```python
from build123d import *

# Parameters (mm, degrees)
SKETCH13_R          = 2.5
SKETCH13_R_2        = 1.5
SKETCH13_W          = 0.45
SKETCH13_H          = 1.7
BOSS_EXTRUDE1_DEPTH = 1.6


with BuildPart() as part:
    # Sketch13 → Boss-Extrude1 (new body)
    # profile 1 of 5: a face of its own
    with BuildSketch(Plane.XY):
        with BuildLine():
            Line((115.98540719, 133.738694526), (115.45540719, 133.738694526))
            ThreePointArc((115.45540719, 133.738694526), (111.919873284, 132.274228432), (110.45540719, 128.738694526))
            Line((110.45540719, 128.738694526), (110.45540719, 123.738694526))
            Line((110.45540719, 123.738694526), (110.45540719, 118.738694526))
            ThreePointArc((110.45540719, 118.738694526), (111.582423844, 115.576416866), (114.45540719, 113.83971504))
            Line((114.45540719, 113.83971504), (114.45540719, 120.238694526))
            Line((114.45540719, 120.238694526), (126.45540719, 120.238694526))
            Line((126.45540719, 120.238694526), (126.45540719, 113.83971504))
            ThreePointArc((126.45540719, 113.83971504), (129.328390536, 115.576416866), (130.45540719, 118.738694526))
            Line((130.45540719, 118.738694526), (130.45540719, 123.738694526))
            Line((130.45540719, 123.738694526), (130.45540719, 128.738694526))
            ThreePointArc((130.45540719, 128.738694526), (128.990941096, 132.274228432), (125.45540719, 133.738694526))
            Line((125.45540719, 133.738694526), (124.92540719, 133.738694526))
            Line((124.92540719, 133.738694526), (124.92540719, 127.388694526))
            Line((124.92540719, 127.388694526), (115.98540719, 127.388694526))
            Line((115.98540719, 127.388694526), (115.98540719, 131.288694526))
            Line((115.98540719, 131.288694526), (115.53540719, 131.288694526))
            Line((115.53540719, 131.288694526), (115.53540719, 132.988694526))
            Line((115.53540719, 132.988694526), (115.98540719, 132.988694526))
            Line((115.98540719, 132.988694526), (115.98540719, 133.738694526))
        make_face()
        with BuildLine():
            ThreePointArc((115.45540719, 123.738694526), (112.95540719, 121.238694526), (110.45540719, 123.738694526))
            ThreePointArc((110.45540719, 123.738694526), (112.95540719, 126.238694526), (115.45540719, 123.738694526))
        make_face(mode=Mode.SUBTRACT)
        with Locations((127.95540719, 123.738694526)):
            Circle(SKETCH13_R, mode=Mode.SUBTRACT)
    # profile 2 of 5: a face of its own
    with BuildSketch(Plane.XY):
        with Locations((112.95540719, 123.738694526)):
            Circle(SKETCH13_R)
        with Locations((112.95540719, 123.738694526)):
            Circle(SKETCH13_R_2, mode=Mode.SUBTRACT)
    # profile 3 of 5: a face of its own
    with BuildSketch(Plane.XY):
        with Locations((127.95540719, 123.738694526)):
            Circle(SKETCH13_R)
        with Locations((127.95540719, 123.738694526)):
            Circle(SKETCH13_R_2, mode=Mode.SUBTRACT)
    # profile 4 of 5: a face of its own
    with BuildSketch(Plane.XY):
        with BuildLine():
            Line((114.45540719, 120.238694526), (114.45540719, 113.83971504))
            ThreePointArc((114.45540719, 113.83971504), (114.95286238, 113.764013761), (115.45540719, 113.738694526))
            Line((115.45540719, 113.738694526), (125.45540719, 113.738694526))
            ThreePointArc((125.45540719, 113.738694526), (125.957952, 113.764013761), (126.45540719, 113.83971504))
            Line((126.45540719, 113.83971504), (126.45540719, 120.238694526))
            Line((126.45540719, 120.238694526), (114.45540719, 120.238694526))
        make_face()
    # profile 5 of 5: a face of its own
    with BuildSketch(Plane.XY):
        with Locations((115.76040719, 132.138694526)):
            Rectangle(SKETCH13_W, SKETCH13_H)
    extrude(amount=BOSS_EXTRUDE1_DEPTH)


solid = part.part
```
The listing builds one solid part. Answer for the finished solid, in the listing's coordinates (mm). A direction names the side the tool comes from. Round coordinates to 2 decimals unless told otherwise and drop trailing zeros. Loops run counter-clockwise (first coordinate to the right, second up) from the corner with the lowest first, then second, coordinate; pieces in that order, holes last. Notation, with made-up numbers: (75, -24.5) - (83, -24.5) arc R21 cw to (83, 5.5) - close; hole circle Ø4 at (14, 18.25). An arc over 180 degrees is marked (long way). Return JSON: item names as keys, results as strings. Group by question number.
1. The part is cut by section B-B on x = 129. Determine the outline of the cut face in (y, z), then the cut area to 3 significant figures.
2. Consider probe 1 along Y at (x, z) = (120.25, 0.35); probe 2 along X at (y, z) = (132.75, 1.1); probe 3 along X at (y, z) = (131.25, 1.3). Determine where each line is inside the solid, lowest interval first.
3. Which of the six approach directions +Z, -Z, +X, -X, +Y, -Y give full straight-line access (tool end or side, diameter ignored) to faces 1 (the cylindrical face through (113.762, 125.004, 0.789)), 2 (the flat face through (124.925, 131, 1))?
4. The part is cut by section D-D on x = 118.75. Determine the outline of the cut face in (y, z).
5. The part is cut by section C-C on y = 130.25. Determine the outline of the cut face in (x, z).
6. Each of these flat-tipped pins is pushed along its axis until it touches: P1, Ø0.5, axis at x = 121.5, z = 0.5, coming from the +Y side; P2, Ø1.8, axis at x = 112.96, y = 123.74, coming from the +Z side. Where does it stop, or does it pass through?
7. The mould has two halves that part along X. Classify faces 3 (the cylindrical face through (129.03, 132.235, 0.789)), 4 (the flat face through (120, 113.739, 1)), 5 (the flat face through (115.985, 131, 1)): pulls with the +X half, pulls with the -X half, needs draft (parallel to the pull), parting line crosses it, or undercut.
8. The part is cut by section A-A on z = 0.3. Determine the outline of the cut face in (x, y), then the cut area to 3 significant figures.
Resolved:
{
 "1": {"outline": "(115.21, 0) - (122.66, 0) - (122.66, 1.6) - (115.21, 1.6) - close; (124.82, 0) - (132.27, 0) - (132.27, 1.6) - (124.82, 1.6) - close", "area": "23.8 mm²"},
 "2": {"probe 1": "y = 113.74 to 127.39", "probe 2": "x = 112.47 to 115.99, 124.93 to 128.44", "probe 3": "x = 111.13 to 115.99, 124.93 to 129.78"},
 "3": {"face 1": "+Z, -Z", "face 2": "+Z, -Z, +Y"},
 "4": {"outline": "(113.74, 0) - (127.39, 0) - (127.39, 1.6) - (113.74, 1.6) - close"},
 "5": {"outline": "(110.69, 0) - (115.99, 0) - (115.99, 1.6) - (110.69, 1.6) - close; (124.93, 0) - (130.22, 0) - (130.22, 1.6) - (124.93, 1.6) - close"},
 "6": {"P1": "stops at y = 127.39", "P2": "passes through"},
 "7": {"face 3": "pulls with the +X half", "face 4": "needs draft", "face 5": "undercut"},
 "8": {"outline": "(110.46, 118.74) arc R5 ccw to (115.46, 113.74) - (125.46, 113.74) arc R5 ccw to (130.46, 118.74) - (130.46, 128.74) arc R5 ccw to (125.46, 133.74) - (124.93, 133.74) - (124.93, 127.39) - (115.99, 127.39) - (115.99, 133.74) - (115.46, 133.74) arc R5 ccw to (110.46, 128.74) - close; hole circle Ø3 at (112.96, 123.74); hole circle Ø3 at (127.96, 123.74)", "area": "308 mm²"}
}
